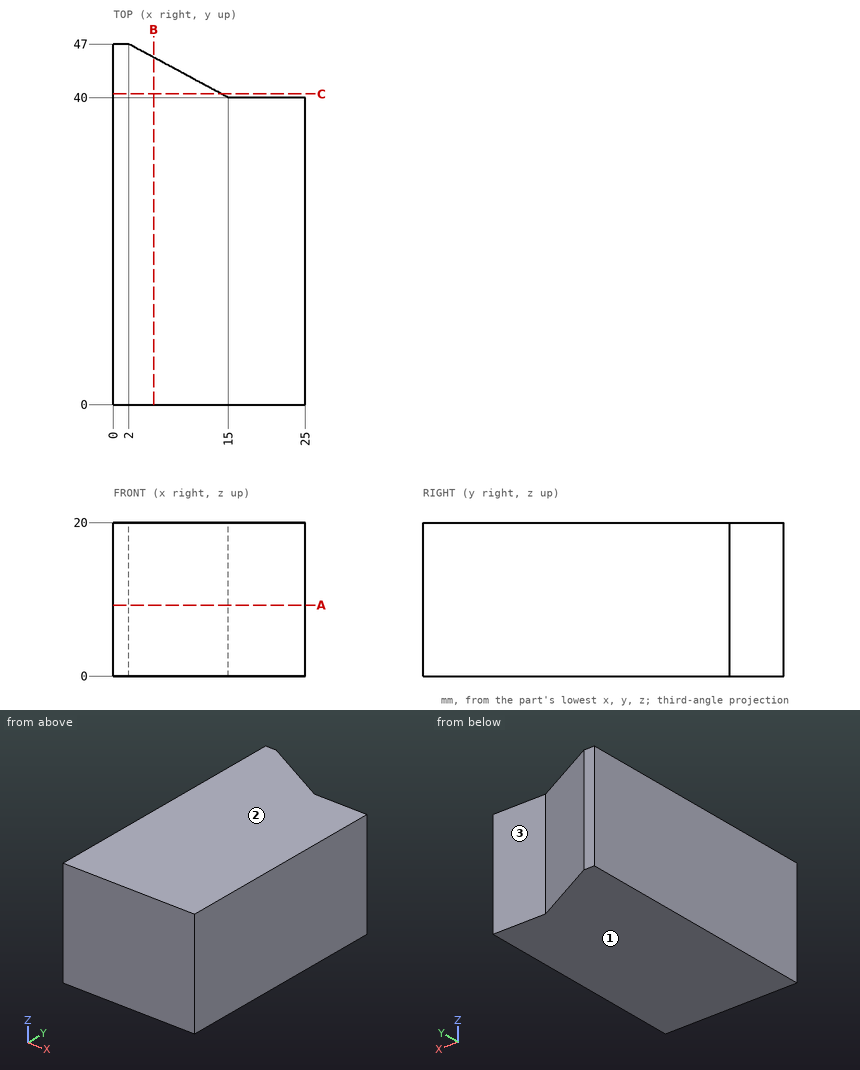
Check sheet for the drawn part. Datum: minimum x, y, z corner. Units: mm. Coordinates: 2 decimals unless noted, no trailing zeros. Loops run counter-clockwise (first coordinate to the right, second up) from the corner with the lowest first, then second, coordinate; pieces in that order, holes last. Notation, with made-up numbers: (39.5, 62.25) -> (95.5, 62.25) arc R5 cw to (95.5, 67.25) -> close; hole circle Ø1 at (17.25, 51.25). An arc over 180 degrees is marked (long way). Answer in a Markdown table with one row per item.
1) Section check B-B (x = 5.25). Record the cut outline in (y, z), and give its area (3 significant figures).
The answers:
| item | result |
|---|---|
| outline | (0, 0) -> (45.25, 0) -> (45.25, 20) -> (0, 20) -> close |
| area | 905 mm2 |
2) Section check C-C (y = 40.5). Record the cut outline in (x, z), and give its area (3 significant figures).
The answers:
| item | result |
|---|---|
| outline | (0, 0) -> (14.07, 0) -> (14.07, 20) -> (0, 20) -> close |
| area | 281 mm2 |
3) Depth check by flat-ended pin: P1, Ø2, axis at x = 11, z = 9.5, coming from the -Y side; P2, Ø5, axis at x = 22, z = 12.5, coming from the +Y side; P3, Ø8, axis at x = 13, z = 7, coming from the +Y side. Enter the tip coordinate at first touch or a pass-through.
The answers:
| item | result |
|---|---|
| P1 | stops at y = 0 |
| P2 | stops at y = 40 |
| P3 | stops at y = 43.23 |
4) Scan lines: line 1 along Y through (x, z) = (15.5, 16); line 2 along Y through (x, z) = (3.5, 3); line 3 along X through (y, z) = (43.5, 17.25). Record each from-to range of solid material in increasing order. Write a range as from..to.
The answers:
| item | result |
|---|---|
| line 1 | y = 0..40 |
| line 2 | y = 0..46.19 |
| line 3 | x = 0..8.5 |
5) Section check A-A (z = 9.25). Record the cut outline in (x, y), and give its area (3 significant figures).
The answers:
| item | result |
|---|---|
| outline | (0, 0) -> (25, 0) -> (25, 40) -> (15, 40) -> (2, 47) -> (0, 47) -> close |
| area | 1,060 mm2 |
6) Draft check along Z on the marked faces 1, 2 and 3. Enter one of: released by +Z, released by -Z, zero draft, split by the parting line, or undercut.
The answers:
| item | result |
|---|---|
| face 1 | released by -Z |
| face 2 | released by +Z |
| face 3 | zero draft |
